```python
from build123d import *

# Parameters (mm, degrees)
F1_DEPTH  = 1.7
F2_W      = 18.7
F2_H      = 20.3
F3_DEPTH  = 3.4
F4_W      = 5
F4_H      = 7.3
F5_DEPTH  = 3.3
F4_W_2    = 5.5
F4_H_2    = 9.5
F4_W_3    = 8.7
F4_H_3    = 4.3
F4_R      = 3.1
F6_DEPTH  = 2.5
F7_W      = 6.7
F7_H      = 6.7
F8_DEPTH  = 1.6
F9_R      = 3.1
F10_DEPTH = 8.4


with BuildPart() as f1:
    # F0 (on Top) → F1 (new body)
    with BuildSketch(Plane.XY):
        Polygon((-10.15, -14.5), (10.15, -14.5), (10.15, 11.5), (-0.55, 11.5), (-0.55, 14.5), (-10.15, 14.5), align=None)
    extrude(amount=F1_DEPTH)

    # F2 (on face) → F3 (join)
    with BuildSketch(Plane.XY.offset(1.7)):
        Rectangle(F2_W, F2_H)
    extrude(amount=F3_DEPTH)

    # F4 (on face) → F5 (join)
    with BuildSketch(Plane(origin=(0, 0, 0), x_dir=(1, 0, 0), z_dir=(0, 0, -1))):
        with Locations((-7.65, 9.057866)):
            Rectangle(F4_W, F4_H)
    extrude(amount=F5_DEPTH)

    # F4 (on face) → F6 (join)
    with BuildSketch(Plane(origin=(0, 0, 0), x_dir=(1, 0, 0), z_dir=(0, 0, -1))):
        with Locations((-3.290825, -1.773557)):
            Rectangle(F4_W_2, F4_H_2)
        with Locations((5.408567, -7.397804)):
            Rectangle(F4_W_3, F4_H_3)
        with Locations((6.664579, 8.933897)):
            Circle(F4_R)
    extrude(amount=F6_DEPTH)

    # F7 (on face) → F8 (join)
    with BuildSketch(Plane(origin=(0, 14.5, 0), x_dir=(-1, 0, 0), z_dir=(0, 1, 0))):
        with Locations((5.3, 2.35)):
            Rectangle(F7_W, F7_H)
    extrude(amount=F8_DEPTH)

    # F9 (on face) → F10 (join)
    with BuildSketch(Plane(origin=(0, 16.1, 0), x_dir=(-1, 0, 0), z_dir=(0, 1, 0))):
        with Locations((5.3, 2.35)):
            Circle(F9_R)
    extrude(amount=F10_DEPTH)


solid = f1.part
```
Could you check a few things on this model? Use its own coordinates, in mm. A direction names the side the tool comes from. Give positions to 0.01 mm unless a question says otherwise; leave off trailing zeros. Write each loop counter-clockwise with the first axis right and the second up, starting at its lowest first coordinate (ties: lowest second). Pieces come first, ordered by that corner, then holes. Notation, with made-up numbers: (62.5, -29) - (76.5, -29) arc R26 ccw to (76.5, -14) - close; hole circle Ø2 at (56, 38). An arc over 180 degrees is marked (long way). One line per item, written item: value. Start each with the question number.
Item 1: I'm going to push flat-ended pins straight in: pin 1 (3.5 mm diameter, centred on x = 6.5, y = 7.5, fed in from -Z); pin 2 (1 mm diameter, centred on y = -8, z = -1, fed in from +X); pin 3 (1.6 mm diameter, centred on x = -7.5, z = -1.5, fed in from +Y); pin 4 (4.5 mm diameter, centred on x = -5, z = 3.5, fed in from -Y). Where does each tip first touch, or does it pass through?
Item 2: Which directions (+Z, -Z, +X, -X, +Y, -Y) give clear straight access to the entire face, cutting with the end or side of a thin tool? Please do faces 4 (the face through (3.568, -9.07, -1.232)), 5 (the face through (-0.55, 13, 1)), 6 (the face through (0, 10.15, 3)), 7 (the face through (-3, -2.976, -1)).
Item 3: Imagine slicing it at C-C, the plane x = 2.25. List the corners of the cut face in (y, z) for me, and give its area (3 significant figures).
Item 4: Imagine slicing it at B-B, the plane y = 2. List the corners of the cut face in (x, z) for me.
Item 5: If we mould it in two halves opening along Y, with no side actions, what happens to faces 1 (the face through (-10.15, -3, 0.3)), 2 (the face through (-8, -12.708, -2)), 3 (the face through (-5, 14.5, 4))? For each: +Y half, -Y half, draft (parallel to the pull), parting line (faces both ways), or undercut.
Item 6: Please list where these lines run through material, in increasing order: line 1 (Y direction, x = -7.5, z = 4.75); line 2 (Y direction, x = -3.5, z = 2); line 3 (Z direction, x = -6.75, y = 8). Write a range as from..to.
Item 7: Imagine slicing it at A-A, the plane z = 2.35. List the corners of the cut face in (x, y) for me.
Item 8: Imagine slicing it at D-D, the plane x = -4.25. List the corners of the cut face in (y, z) for me, and give its area (3 significant figures).
Geometry says:
1. pin 1: z = -2.5
1. pin 2: x = 9.73
1. pin 3: y = 16.1
1. pin 4: y = -14.5
2. face 4: -Z
2. face 5: +Z, -Z, +X, +Y
2. face 6: +Z, +X, -X
2. face 7: -Z, +X, -X
3. outline: (-14.5, 0) - (5.25, 0) - (5.25, -2.5) - (9.55, -2.5) - (9.55, 0) - (11.5, 0) - (11.5, 1.7) - (10.15, 1.7) - (10.15, 5.1) - (-10.15, 5.1) - (-10.15, 1.7) - (-14.5, 1.7) - close
3. area: 124 mm^2
4. outline: (-10.15, 0) - (-6.04, 0) - (-6.04, -2.5) - (-0.54, -2.5) - (-0.54, 0) - (10.15, 0) - (10.15, 1.7) - (9.35, 1.7) - (9.35, 5.1) - (-9.35, 5.1) - (-9.35, 1.7) - (-10.15, 1.7) - close
5. face 1: draft
5. face 2: -Y half
5. face 3: undercut
6. line 1: -10.15..10.15, 14.5..16.1
6. line 2: -10.15..10.15, 14.5..24.5
6. line 3: 0..5.1
7. outline: (-9.35, -10.15) - (9.35, -10.15) - (9.35, 10.15) - (-9.35, 10.15) - close; (-8.65, 14.5) - (-1.95, 14.5) - (-1.95, 16.1) - (-2.2, 16.1) - (-2.2, 24.5) - (-8.4, 24.5) - (-8.4, 16.1) - (-8.65, 16.1) - close
8. outline: (-14.5, 0) - (-2.98, 0) - (-2.98, -2.5) - (6.52, -2.5) - (6.52, 0) - (14.5, 0) - (14.5, -1) - (16.1, -1) - (16.1, -0.57) - (24.5, -0.57) - (24.5, 5.27) - (16.1, 5.27) - (16.1, 5.7) - (14.5, 5.7) - (14.5, 1.7) - (10.15, 1.7) - (10.15, 5.1) - (-10.15, 5.1) - (-10.15, 1.7) - (-14.5, 1.7) - close
8. area: 202 mm^2
